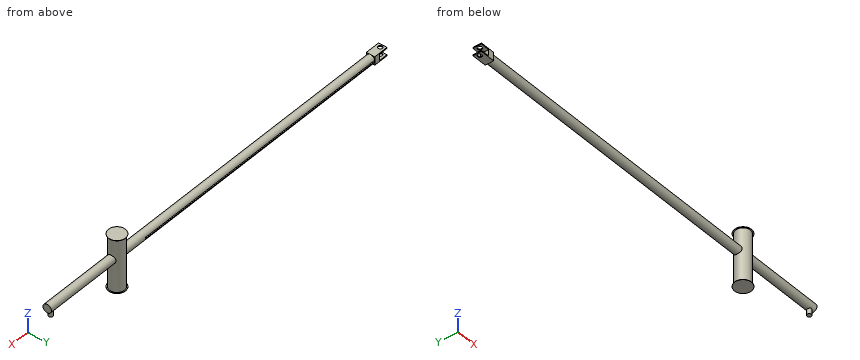
```python
from build123d import *

# Parameters (mm, degrees)
SKETCH_1_R           = 2
EXTRUDE_1_DEPTH      = 192.4
SKETCH_2_R           = 1
EXTRUDE_2_DEPTH      = 4.5
SKETCH_3_R           = 3.5
EXTRUDE_3_DEPTH      = 10
EXTRUDE_3_DEPTH_BACK = 15.1
SKETCH_4_R           = 4
EXTRUDE_4_DEPTH      = 0.1
SKETCH_5_R           = 4
EXTRUDE_5_DEPTH      = 0.1
SKETCH_6_W           = 7
SKETCH_6_H           = 4
EXTRUDE_6_DEPTH      = 2
SKETCH_7_W           = 4.2
SKETCH_7_H           = 3
CUT_EXTRUDE_1_DEPTH  = 2
SKETCH_8_R           = 1
CUT_EXTRUDE_2_DEPTH  = 2
SKETCH_9_W           = 131.4
SKETCH_9_H           = 0.6
CUT_EXTRUDE_3_DEPTH  = 0.5


with BuildPart() as part:
    # 草图1 → 凸台-拉伸1 (new body)
    with BuildSketch(Plane(origin=(0, 0, 0), x_dir=(0, 0, -1), z_dir=(1, 0, 0))):
        Circle(SKETCH_1_R)
    extrude(amount=EXTRUDE_1_DEPTH)

    # 草图2 → 凸台-拉伸2 (add)
    with BuildSketch(Plane.XY):
        with Locations((2, 0)):
            Circle(SKETCH_2_R)
    extrude(amount=-EXTRUDE_2_DEPTH)

    # 草图3 → 凸台-拉伸3 (add, two sides)
    with BuildSketch(Plane.XY) as extrude_3_sk:
        with Locations((40, 0)):
            Circle(SKETCH_3_R)
    extrude(amount=EXTRUDE_3_DEPTH)
    extrude(extrude_3_sk.sketch, amount=-EXTRUDE_3_DEPTH_BACK)

    # 草图4 → 凸台-拉伸4 (add)
    with BuildSketch(Plane.XY.offset(10)):
        with Locations((40, 0)):
            Circle(SKETCH_4_R)
    extrude(amount=-EXTRUDE_4_DEPTH)

    # 草图5 → 凸台-拉伸5 (add)
    with BuildSketch(Plane(origin=(0, 0, -15.1), x_dir=(-1, 0, 0), z_dir=(0, 0, -1))):
        with Locations((-40, 0)):
            Circle(SKETCH_5_R)
    extrude(amount=EXTRUDE_5_DEPTH)

    # 草图6 → 凸台-拉伸6 (add, symmetric)
    with BuildSketch(Plane(origin=(0, 0, 0), x_dir=(1, 0, 0), z_dir=(0, 1, 0))):
        with Locations((188.9, 0)):
            Rectangle(SKETCH_6_W, SKETCH_6_H)
    extrude(amount=EXTRUDE_6_DEPTH, both=True)

    # 草图7 → 切除-拉伸1 (cut, symmetric)
    with BuildSketch(Plane(origin=(0, 0, 0), x_dir=(1, 0, 0), z_dir=(0, 1, 0))):
        with Locations((190.3, 0)):
            Rectangle(SKETCH_7_W, SKETCH_7_H)
    extrude(amount=CUT_EXTRUDE_1_DEPTH, both=True, mode=Mode.SUBTRACT)

    # 草图8 → 切除-拉伸2 (cut, symmetric)
    with BuildSketch(Plane.XY):
        with Locations((190.9, 0)):
            Circle(SKETCH_8_R)
    extrude(amount=CUT_EXTRUDE_2_DEPTH, both=True, mode=Mode.SUBTRACT)

    # 草图9 → 切除-拉伸3 (cut)
    with BuildSketch(Plane(origin=(0, 2, 0), x_dir=(1, 0, 0), z_dir=(0, 1, 0))):
        with Locations((119.7, 0)):
            Rectangle(SKETCH_9_W, SKETCH_9_H)
    extrude(amount=-CUT_EXTRUDE_3_DEPTH, mode=Mode.SUBTRACT)


with BuildPart() as body_2:
    # 镜向1: mirrored copy
    add(part.part.mirror(Plane(origin=(0, 0, 0), x_dir=(0, 0, 1), z_dir=(1, 0, 0))))


solid = body_2.part
```
Here's how the part is built. I have some questions about the finished solid (model axes, mm). Round coordinates to 2 decimals unless told otherwise and drop trailing zeros. Write each loop counter-clockwise with the first axis right and the second up, starting at its lowest first coordinate (ties: lowest second). Pieces come first, ordered by that corner, then holes.
Q1. If we section it at B-B on x = -86: Write out the boundary of the cut face in (y, z), plus the area to 3 significant figures.
Q2. Please list where these lines run through material, in increasing order: probe 1 along Y at (x, z) = (-190.9, 1.85); probe 2 along X at (y, z) = (-2, -10.5); probe 3 along X at (y, z) = (0, -6.75).
Q3. Will these pins go through, and if not, where does the flat tip stop? P1, Ø1.2, axis at x = -191, y = -0.5, coming from the +Z side; P2, Ø3, axis at x = -190.5, y = 0.5, coming from the -Z side; P3, Ø4.5, axis at x = -189.5, z = 0, coming from the -Y side.
Q4. If we section it at A-A on x = -40: Write out the boundary of the cut face in (y, z).
Answer below:
1. outline: (1.5, -0.3) - (1.5, 0.3) - (1.98, 0.3) arc R2 ccw (long way) to (1.98, -0.3) - close
1. area: 12.3 mm2
2. probe 1: y = -2 to -1, 1 to 2
2. probe 2: x = -42.87 to -37.13
2. probe 3: x = -43.5 to -36.5
3. P1: stops at z = 2
3. P2: stops at z = -2
3. P3: stops at y = -2
4. outline: (-4, -15.2) - (4, -15.2) - (4, -15.1) - (3.5, -15.1) - (3.5, 9.9) - (4, 9.9) - (4, 10) - (-4, 10) - (-4, 9.9) - (-3.5, 9.9) - (-3.5, -15.1) - (-4, -15.1) - close
